Verification items for the finished model (mm, model axes). A direction names the side the tool comes from. Give positions to 0.01 mm unless a question says otherwise; leave off trailing zeros. Order: outer loops, then holes, each group sorted by start corner. A loop starts at its lowest first (then second) coordinate and runs counter-clockwise, first axis right, second up. Notation, with made-up numbers: (-7.75, -7.5) -> (5.25, -7.5) arc R17 cw to (5.25, 3.5) -> close; hole circle Ø5 at (-7.75, 89). An arc over 180 degrees is marked (long way). One line per question, with ' | ' between items. Start each with the question number.
Q1. Section check B-B on z = -12. Record the cut outline in (x, y), plus the area to 3 significant figures.
Q2. Mould release check, pull along Z, two halves, no side actions. Record for faces 4 (the cylindrical face through (-14.985, 171.479, 0.66)), 5 (the flat face through (9, 2, 1.5)), 6 (the cylindrical face through (8.894, 171.479, 6.066)): released by +Z, released by -Z, zero draft, split by the parting line, or undercut.
Q3. Go/stop test with flat-tipped pins: pin 1 (3.5 mm diameter, centred on x = 8.5, y = 2.5, fed in from -Z); pin 2 (2 mm diameter, centred on y = 32.5, z = -6.5, fed in from -X); pin 3 (8 mm diameter, centred on x = -0.5, y = 36, fed in from -Z). Record where each tip stops, or that it passes through.
Q4. Section check A-A on x = 0. Record the cut outline in (y, z).
Q5. Section check C-C on y = 39.5. Record the cut outline in (x, z), plus the area to 3 significant figures.
Q6. Section check D-D on z = 0. Record the cut outline in (x, y), plus the area to 3 significant figures.
Q7. Material ranges on probe 1 along X at (y, z) = (171, 6); probe 2 along Z at (x, y) = (0, 52); probe 3 along Y at (x, z) = (-12.25, 5.5), recorded low to high. Write a range as [from, to].
Q8. Access from +Z, -Z, +X, -X, +Y, -Y to the whole of each face (thin tool, end or side, straight path). Record for faces 1 (the flat face through (10.5, 2, 0)), 2 (the flat face through (9, 3, -1.5)), 3 (the flat face through (-4, 173, -4)).
Autodesk Inventor part; units mm, degrees
ref_plane "Work Plane1" through (7.5, 0, 0) normal (1, 0, 0) x (0, 1, 0)
ref_plane "XZ Plane" through (0, 0, 0) normal (0, 1, 0) x (-1, 0, 0)
ref_plane "XY Plane" through (0, 0, 0) normal (0, 0, 1) x (1, 0, 0)
sketch "Sketch1" plane through (0, 0, 0) normal (0, 1, 0) x (-1, 0, 0)
  circle A0 centre (0, 0) radius 7.5
  circle A1 centre (0, 0) radius 5
  dimension "d0" = 2.5
  dimension "d1" = 15
extrude "Extrusion1" add sketch "Sketch1" along normal blind 170
ref_plane "Work Plane1" through (7.5, 0, 0) normal (1, 0, 0) x (0, 1, 0)
sketch "Sketch2" plane through (7.5, 0, 0) normal (1, 0, 0) x (0, 1, 0)
  line L0 (0, -7.5) -> (0, 7.5)
  line L1 (0, -1.5) -> (0, 1.5)
  line L2 (0, 1.5) -> (5, 1.5)
  line L3 (5, 1.5) -> (5, -1.5)
  line L4 (5, -1.5) -> (0, -1.5)
  point P0 (0, 0)
  dimension "d4" = 1.5
  dimension "d5" = 1.5
  dimension "d6" = 5
extrude "Extrusion2" add sketch "Sketch2" along normal blind 3 and the other way blind 1.5
sketch "Sketch4" plane through (0, 170, 0) normal (0, 1, 0) x (1, 0, 0)
  circle A0 centre (0, 0) radius 15
  circle A1 centre (0, 0) radius 5
  circle A2 centre (0, 12) radius 1.5
  circle A3 centre (-10.3923, -6) radius 1.5
  circle A4 centre (10.3923, -6) radius 1.5
  dimension "d11" = 30
  dimension "d12" = 12
  dimension "d13" = 3
  dimension "d16" = 360
extrude "Extrusion3" add sketch "Sketch4" along normal blind 3
properties part number "15"
Filled in:
1) outline: (-9, 170) -> (-1.5, 170) -> (-1.5, 173) -> (-9, 173) -> close; (1.5, 170) -> (9, 170) -> (9, 173) -> (1.5, 173) -> close | area: 45.0 mm²
2) face 4: split by the parting line | face 5: released by +Z | face 6: undercut
3) pin 1: z = -3.27 | pin 2: x = -5.1 | pin 3: z = -7.5
4) outline: (0, -7.5) -> (170, -7.5) -> (170, -10.5) -> (173, -10.5) -> (173, -5) -> (0, -5) -> close; (0, 5) -> (173, 5) -> (173, 15) -> (170, 15) -> (170, 7.5) -> (0, 7.5) -> close; (170, -15) -> (173, -15) -> (173, -13.5) -> (170, -13.5) -> close
5) outline: circle Ø15 at (0, 0); hole circle Ø10 at (0, 0) | area: 98.2 mm²
6) outline: (-15, 170) -> (-7.5, 170) -> (-7.5, 0) -> (-5, 0) -> (-5, 173) -> (-15, 173) -> close; (5, 0) -> (10.5, 0) -> (10.5, 5) -> (7.5, 5) -> (7.5, 170) -> (15, 170) -> (15, 173) -> (5, 173) -> close | area: 925 mm²
7) probe 1: [-13.75, -11.89], [-8.89, 8.89], [11.89, 13.75] | probe 2: [-7.5, -5], [5, 7.5] | probe 3: [170, 173]
8) face 1: +Z, -Z, +X, -Y | face 2: -Z, +X, -Y | face 3: +Z, -Z, +X, -X, +Y
